from build123d import *

# Parameters (mm, degrees)
BOSS_EXTRUDE1_DEPTH = 10
SKETCH2_R           = 11.75
SKETCH2_R_2         = 1.45
MOTOR_DEPTH         = 57.789083458
SCREW_DEPTH         = 57.789083458
SKETCH4_W           = 25
SKETCH4_H           = 5
CUT_EXTRUDE3_DEPTH  = 57.789083458


with BuildPart() as part:
    # Sketch1 → Boss-Extrude1 (new body)
    with BuildSketch(Plane.XY):
        Polygon((0, 0), (0, -5), (-10, -5), (-10, -15), (0, -15), (0, -35), (-10, -35), (-10, -45), (0, -45), (0, -50), (25, -50), (25, 0), align=None)
    extrude(amount=BOSS_EXTRUDE1_DEPTH)

    # Sketch2 → motor (cut, through all)
    with BuildSketch(Plane.XY.offset(10)):
        with Locations((25, -21)):
            Circle(SKETCH2_R)
        with Locations((9.5, -5.5)):
            Circle(SKETCH2_R_2)
        with Locations(Location((9.5, -36.5, 0), (0, 0, 180))):
            Circle(SKETCH2_R_2)
    extrude(amount=-MOTOR_DEPTH, mode=Mode.SUBTRACT)

    # Sketch3 → screw (cut, through all)
    with BuildSketch(Plane.XY.offset(10)):
        with BuildLine():
            Line((0, -26.55), (0, -23.45))
            Line((0, -23.45), (4.5, -23.45))
            Line((4.5, -23.45), (4.5, -22.65))
            ThreePointArc((4.5, -22.65), (4.646446609, -22.296446609), (5, -22.15))
            Line((5, -22.15), (7.5, -22.15))
            ThreePointArc((7.5, -22.15), (7.853553391, -22.296446609), (8, -22.65))
            Line((8, -22.65), (8, -23.45))
            Line((8, -23.45), (10.5, -23.45))
            Line((10.5, -23.45), (10.5, -26.55))
            Line((10.5, -26.55), (8, -26.55))
            Line((8, -26.55), (8, -27.35))
            ThreePointArc((8, -27.35), (7.853553391, -27.703553391), (7.5, -27.85))
            Line((7.5, -27.85), (5, -27.85))
            ThreePointArc((5, -27.85), (4.646446609, -27.703553391), (4.5, -27.35))
            Line((4.5, -27.35), (4.5, -26.55))
            Line((4.5, -26.55), (0, -26.55))
        make_face()
    extrude(amount=-SCREW_DEPTH, mode=Mode.SUBTRACT)

    # Sketch4 → Cut-Extrude3 (cut, through all)
    with BuildSketch(Plane.XY.offset(10)):
        with Locations((12.5, -47.5)):
            Rectangle(SKETCH4_W, SKETCH4_H)
        Polygon((0, -5), (5, 0), (0, 0), align=None)
    extrude(amount=-CUT_EXTRUDE3_DEPTH, mode=Mode.SUBTRACT)


solid = part.part
Input: part model. Units: mm. Frame: model coordinates. A direction names the side the tool comes from. Give positions to 0.01 mm unless a question says otherwise; leave off trailing zeros. Order: outer loops, then holes, each group sorted by start corner. A loop starts at its lowest first (then second) coordinate and runs counter-clockwise, first axis right, second up.
Q1. Section A-A on z = 8.75. State how many separate pieces and enclosed holes the cut face has, and give its area (3 significant figures).
Checked values:
separate pieces: 1
enclosed holes: 2
area: 1,040 mm2
Q2. Ray query, probe 1 along Y at (x, z) = (9.5, 5); probe 2 along X at (y, z) = (-36.5, 4.75); probe 3 along Y at (x, z) = (5.5, 7). Return the intervals inside material, ascending.
Checked values:
probe 1: y = -45 to -37.95, -35.05 to -26.55, -23.45 to -6.95, -4.05 to 0
probe 2: x = -10 to 8.05, 10.95 to 25
probe 3: y = -45 to -27.85, -22.15 to 0
Q3. Section D-D on x = 9.5. Output: boundary loops of the cut face in (y, z).
Checked values:
outline: (-45, 0) - (-37.95, 0) - (-37.95, 10) - (-45, 10) - close; (-35.05, 0) - (-26.55, 0) - (-26.55, 10) - (-35.05, 10) - close; (-23.45, 0) - (-6.95, 0) - (-6.95, 10) - (-23.45, 10) - close; (-4.05, 0) - (0, 0) - (0, 10) - (-4.05, 10) - close
Q4. Section B-B on y = -36.5. Output: boundary loops of the cut face in (x, z), and give its area (3 significant figures).
Checked values:
outline: (-10, 0) - (8.05, 0) - (8.05, 10) - (-10, 10) - close; (10.95, 0) - (25, 0) - (25, 10) - (10.95, 10) - close
area: 321 mm2
Q5. Set-up query: faces 1 (the flat face through (25, -5, 5)), 2 (the flat face through (2, -26.55, 5)), 3 (the flat face through (6, -22.15, 5)), 4 (the cylindrical face through (13.253, -20.742, 5.07)), 5 (the flat face through (-5, -5, 5)). Return all of +Z, -Z, +X, -X, +Y, -Y with unobstructed straight access to the full face (end or side cutting, diameter ignored); none if empty.
Checked values:
face 1: +Z, -Z, +X, +Y, -Y
face 2: +Z, -Z, -X
face 3: +Z, -Z
face 4: +Z, -Z, +X
face 5: +Z, -Z, -X, +Y
Q6. Draft query along Y for faces 6 (the flat face through (15, 0, 5)), 7 (the flat face through (-5, -15, 5)), 8 (the flat face through (25, -39, 5)), 9 (the flat face through (2, -23.45, 5)). Return one class per face: +Y half, -Y half, draft (parallel to the pull), parting line (faces both ways), or undercut.
Checked values:
face 6: +Y half
face 7: undercut
face 8: draft
face 9: undercut
Q7. Contact query for flat-ended pins moving along their axis: pin 1 Ø3 at (x, z) = (-7, 6.5) entering from +Y; pin 2 Ø3 at (y, z) = (-28, 6) entering from -X; pin 3 Ø5 at (x, z) = (1.5, 2.5) entering from +Y. Output: stop coordinate, or through.
Checked values:
pin 1: stops at y = -5
pin 2: stops at x = 0
pin 3: stops at y = -1
Q8. Section C-C on x = 16.5. Output: boundary loops of the cut face in (y, z).
Checked values:
outline: (-45, 0) - (-29.11, 0) - (-29.11, 10) - (-45, 10) - close; (-12.89, 0) - (0, 0) - (0, 10) - (-12.89, 10) - close
